The model under review builds one solid part; all positions refer to its coordinate system, in mm. A direction names the side the tool comes from. Round coordinates to 2 decimals unless told otherwise and drop trailing zeros. Loops run counter-clockwise (first coordinate to the right, second up) from the corner with the lowest first, then second, coordinate; pieces in that order, holes last. Notation, with made-up numbers: (-10, 68) - (-3, 68) arc R28 cw to (-3, 96) - close; hole circle Ø1 at (39, 15.5). An arc over 180 degrees is marked (long way). Answer as CSV lines item,"result".
from build123d import *

# Parameters (mm, degrees)
F0_R      = 38.1
F0_R_2    = 30.48
F1_DEPTH  = 50.8
F3_W      = 101.6
F3_H      = 203.2
F4_DEPTH  = 12.7
F5_W      = 101.3802451253
F5_H      = 189.2143650602
F6_DEPTH  = 6.35
F8_DEPTH  = 49.784
F9_W      = 81.0602451253
F9_H      = 121.0168540975
F10_DEPTH = 25.4


with BuildPart() as f1:
    # F0 (on Top) → F1 (new body)
    with BuildSketch(Plane.XY):
        Circle(F0_R)
        Circle(F0_R_2, mode=Mode.SUBTRACT)
    extrude(amount=F1_DEPTH)



with BuildPart() as f4:
    # F3 (on offset) → F4 (new body)
    with BuildSketch(Plane.XY.offset(-138.43)):
        with Locations((0, 62.8368258476)):
            Rectangle(F3_W, F3_H)
    extrude(amount=F4_DEPTH)


with BuildPart() as f6:
    # F5 (on face) → F6 (new body)
    with BuildSketch(Plane.XZ.offset(38.7631741524)):
        with Locations((-0.1098774374, -43.8228174699)):
            Rectangle(F5_W, F5_H)
    extrude(amount=-F6_DEPTH)


with BuildPart() as f1_1:
    add(f1.part)

    add(f6.part)  # F8 merges F6
    # F7 (on face) → F8 (join)
    with BuildSketch(Plane.XY.offset(50.7843650602)):
        with BuildLine():
            Line((-37.9473480204, 0), (-50.8, -32.4131741524))
            Line((-50.8, -32.4131741524), (-19.7329005255, -32.4131741524))
            ThreePointArc((-19.7329005255, -32.4131741524), (-33.081811207, -18.5901852881), (-37.9473480204, 0))
        make_face()
        with BuildLine():
            Line((19.7329005255, -32.4131741524), (50.5802451253, -32.4131741524))
            Line((50.5802451253, -32.4131741524), (37.945801456, -0.3425983667))
            ThreePointArc((37.945801456, -0.3425983667), (32.997554809, -18.7393329232), (19.7329005255, -32.4131741524))
        make_face()
    extrude(amount=-F8_DEPTH)

    # F9 (on face) → F10 (cut)
    with BuildSketch(Plane.XZ.offset(38.7631741524)):
        with Locations((-0.1098774374, -65.1476242347)):
            Rectangle(F9_W, F9_H)
    extrude(amount=-F10_DEPTH, mode=Mode.SUBTRACT)



with BuildPart() as f1_2:
    add(f1_1.part)

    add(f4.part)  # F11 merges F4
    # F11: F1 across plane
    add(f1_1.part.mirror(Plane.XZ))


solid = f1_2.part
1. Clearance check with flat-ended pins moving along their axes: pin 1 (5 mm diameter, centred on y = -36, z = -92.5, fed in from +X); pin 2 (8 mm diameter, centred on x = -28, y = 87, fed in from +Z); pin 3 (3 mm diameter, centred on x = -37, z = -7.5, fed in from +Y). State where each tip first meets the part, or that it passes through.
Numbers:
pin 1,"stops at x = 50.58"
pin 2,"stops at z = -125.73"
pin 3,"passes through"
2. Take a section at B-B (z = -118.5). State the section outline as (x, y) points, plus the area to 3 significant figures.
Numbers:
outline,"(-50.8, -38.76) - (-40.64, -38.76) - (-40.64, -32.41) - (-50.8, -32.41) - close; (-50.8, 32.41) - (-40.64, 32.41) - (-40.64, 38.76) - (-50.8, 38.76) - close; (40.42, -38.76) - (50.58, -38.76) - (50.58, -32.41) - (40.42, -32.41) - close; (40.42, 32.41) - (50.58, 32.41) - (50.58, 38.76) - (40.42, 38.76) - close"
area,"258 mm²"
3. Take a section at A-A (x = 0). State how many separate pieces and enclosed holes the cut face has, plus the area to 3 significant figures.
Numbers:
separate pieces,"3"
enclosed holes,"0"
area,"3,480 mm²"
4. Draft analysis for pull direction Y (two halves, no side actions). For faces 4 (the face through (50.58, -36, -39)), 5 (the face through (-26, -17, 0)), 6 (the face through (-1, 164.437, -132)), state which applies: +Y half, -Y half, draft (parallel to the pull), parting line (faces both ways), or undercut.
Numbers:
face 4,"draft"
face 5,"undercut"
face 6,"+Y half"
5. Wall thickness on probe 1 along Y at (x, z) = (0, 16); probe 2 along X at (y, z) = (36.5, -116.5); probe 3 along Y at (x, z) = (10, -0.5): over which ranges is each line inside the solid? List them lowest first.
Numbers:
probe 1,"y = -38.76 to -30.48, 30.48 to 38.76"
probe 2,"x = -50.8 to -40.64, 40.42 to 50.58"
probe 3,"y = -38.76 to -32.41, 32.41 to 38.76"
6. Tool access review of faces 1 (the face through (-38.096, 0.559, 0.822)), 2 (the face through (-44.36, 16.17, 26.24)), 3 (the face through (40.42, 36, -66)): name each direction out of +Z, -Z, +X, -X, +Y, -Y from which nothing blocks a thin tool from reaching the whole face with its end or side.
Numbers:
face 1,"none"
face 2,"+Z, -X"
face 3,"+Y, -Y"
